from build123d import *

# Parameters (mm, degrees)
SKETCH1_R               = 33
BOSS_EXTRUDE1_DEPTH     = 2
SKETCH5_R               = 27
BOSS_EXTRUDE2_DEPTH     = 2
SKETCH7_W               = 35
SKETCH7_H               = 25
CUT_EXTRUDE2_DEPTH      = 2
FILLET5_R               = 2
CUT_EXTRUDE3_DEPTH      = 47.840153715
CUT_EXTRUDE3_DEPTH_BACK = 47.840153715
SKETCH8_W               = 35
SKETCH8_H               = 5
FILLET3_R               = 2
SKETCH6_R               = 2
CUT_EXTRUDE4_DEPTH      = 10


with BuildPart() as part:
    # Sketch1 → Boss-Extrude1 (new body)
    with BuildSketch(Plane(origin=(0, 0, 0), x_dir=(1, 0, 0), z_dir=(0, 1, 0))):
        with Locations(Location((0, 0, 0), (0, 0, 270))):
            Circle(SKETCH1_R)
    extrude(amount=BOSS_EXTRUDE1_DEPTH)

    # Sketch5 → Boss-Extrude2 (add)
    with BuildSketch(Plane.XZ):
        with Locations(Location((0, 0, 0), (0, 0, 270))):
            Circle(SKETCH5_R)
    extrude(amount=BOSS_EXTRUDE2_DEPTH)

    # Sketch7 → Cut-Extrude2 (cut)
    with BuildSketch(Plane(origin=(0, 2, 0), x_dir=(1, 0, 0), z_dir=(0, 1, 0))):
        Rectangle(SKETCH7_W, SKETCH7_H)
    extrude(amount=-CUT_EXTRUDE2_DEPTH, mode=Mode.SUBTRACT)

    # Fillet5
    fillet5_edges = [part.edges().sort_by_distance(p)[0] for p in [
        (0, -2, 27),
    ]]
    fillet(fillet5_edges, radius=FILLET5_R - 0.0001)  # a hair under: the kernel refuses the full size

    # Sketch8 → Cut-Extrude3 (cut, two sides: drawn at the far end of the back side and taken through both)
    with BuildSketch(Plane(origin=(0, 2, 0), x_dir=(1, 0, 0), z_dir=(0, 1, 0)).offset(-CUT_EXTRUDE3_DEPTH_BACK)):
        with Locations((0, -10)):
            Rectangle(SKETCH8_W, SKETCH8_H)
    extrude(amount=CUT_EXTRUDE3_DEPTH + CUT_EXTRUDE3_DEPTH_BACK, mode=Mode.SUBTRACT)

    # Fillet3
    fillet3_edges = [part.edges().sort_by_distance(p)[0] for p in [
        (0, 2, 12.5),
        (-17.5, 2, 0),
        (0, 2, -12.5),
        (17.5, 2, 0),
    ]]
    fillet(fillet3_edges, radius=FILLET3_R - 0.0001)  # a hair under: the kernel refuses the full size

    # Sketch6 → Cut-Extrude4 (cut)
    with BuildSketch(Plane.XZ):
        with BuildLine():
            ThreePointArc((3.5, 32.813869019), (0, 33), (-3.5, 32.813869019))
            Line((-3.5, 32.813869019), (-2.640595233, 27.71772001))
            ThreePointArc((-2.640595233, 27.71772001), (-2.300161408, 27.12037077), (-1.654518359, 26.884010118))
            Line((-1.654518359, 26.884010118), (1.654518359, 26.884010118))
            ThreePointArc((1.654518359, 26.884010118), (2.300161408, 27.12037077), (2.640595233, 27.71772001))
            Line((2.640595233, 27.71772001), (3.5, 32.813869019))
        make_face()
        with BuildLine():
            Line((25.32454728, 11.572037452), (30.167644167, 13.375845596))
            ThreePointArc((30.167644167, 13.375845596), (28.578838325, 16.5), (26.667644167, 19.438023423))
            Line((26.667644167, 19.438023423), (22.683952047, 16.145682558))
            ThreePointArc((22.683952047, 16.145682558), (22.336849342, 15.552183597), (22.454976538, 14.874859989))
            Line((22.454976538, 14.874859989), (24.109494897, 12.009150128))
            ThreePointArc((24.109494897, 12.009150128), (24.637010751, 11.568187173), (25.32454728, 11.572037452))
        make_face()
        with Locations(Location((-15.850338446, 24.880047651, 0), (0, 0, 270))):
            Circle(SKETCH6_R)
        with BuildLine():
            Line((-30.167644167, 13.375845596), (-25.32454728, 11.572037452))
            ThreePointArc((-25.32454728, 11.572037452), (-24.637010751, 11.568187173), (-24.109494897, 12.009150128))
            Line((-24.109494897, 12.009150128), (-22.454976538, 14.874859989))
            ThreePointArc((-22.454976538, 14.874859989), (-22.336849342, 15.552183597), (-22.683952047, 16.145682558))
            Line((-22.683952047, 16.145682558), (-26.667644167, 19.438023423))
            ThreePointArc((-26.667644167, 19.438023423), (-28.578838325, 16.5), (-30.167644167, 13.375845596))
        make_face()
        with BuildLine():
            Line((22.683952047, -16.145682558), (26.667644167, -19.438023423))
            ThreePointArc((26.667644167, -19.438023423), (28.578838325, -16.5), (30.167644167, -13.375845596))
            Line((30.167644167, -13.375845596), (25.32454728, -11.572037452))
            ThreePointArc((25.32454728, -11.572037452), (24.637010751, -11.568187173), (24.109494897, -12.009150128))
            Line((24.109494897, -12.009150128), (22.454976538, -14.874859989))
            ThreePointArc((22.454976538, -14.874859989), (22.336849342, -15.552183597), (22.683952047, -16.145682558))
        make_face()
        with Locations(Location((15.850338446, -24.880047651, 0), (0, 0, 270))):
            Circle(SKETCH6_R)
        with BuildLine():
            Line((-26.667644167, -19.438023423), (-22.683952047, -16.145682558))
            ThreePointArc((-22.683952047, -16.145682558), (-22.336849342, -15.552183597), (-22.454976538, -14.874859989))
            Line((-22.454976538, -14.874859989), (-24.109494897, -12.009150128))
            ThreePointArc((-24.109494897, -12.009150128), (-24.637010751, -11.568187173), (-25.32454728, -11.572037452))
            Line((-25.32454728, -11.572037452), (-30.167644167, -13.375845596))
            ThreePointArc((-30.167644167, -13.375845596), (-28.578838325, -16.5), (-26.667644167, -19.438023423))
        make_face()
        with BuildLine():
            Line((-2.640595233, -27.71772001), (-3.5, -32.813869019))
            ThreePointArc((-3.5, -32.813869019), (0, -33), (3.5, -32.813869019))
            Line((3.5, -32.813869019), (2.640595233, -27.71772001))
            ThreePointArc((2.640595233, -27.71772001), (2.300161408, -27.12037077), (1.654518359, -26.884010118))
            Line((1.654518359, -26.884010118), (-1.654518359, -26.884010118))
            ThreePointArc((-1.654518359, -26.884010118), (-2.300161408, -27.12037077), (-2.640595233, -27.71772001))
        make_face()
    extrude(amount=-CUT_EXTRUDE4_DEPTH, mode=Mode.SUBTRACT)


solid = part.part
Design review of the part built by this model. Coordinates are the model's own, in mm. A direction names the side the tool comes from. Round coordinates to 2 decimals unless told otherwise and drop trailing zeros. Write each loop counter-clockwise with the first axis right and the second up, starting at its lowest first coordinate (ties: lowest second). Pieces come first, ordered by that corner, then holes. Notation, with made-up numbers: (3.5, 75) -> (11.5, 75) arc R11 ccw to (11.5, 96) -> close; hole circle Ø10 at (48.25, 41.5). An arc over 180 degrees is marked (long way). One line per question, with ' | ' between items.
(1) Take a section at D-D, the plane x = -28. State the section outline as (y, z) points, and give its area (3 significant figures).
Result sheet:
outline: (0, -12.57) -> (2, -12.57) -> (2, 12.57) -> (0, 12.57) -> close | area: 50.3 mm2
(2) Draft analysis for pull direction Z (two halves, no side actions). For faces 1 (the flat face through (0, 2, -15)), 2 (the cylindrical face through (16.67, 0.99, -28.48)), 3 (the flat face through (-24.65, 0.99, 17.77)), 4 (the flat face through (0, -1, 7.5)), state which applies: released by +Z, released by -Z, zero draft, split by the parting line, or undercut.
Result sheet:
face 1: zero draft | face 2: released by -Z | face 3: undercut | face 4: undercut
(3) Machinability: for faces 5 (the flat face through (0, 1, -26.884)), 6 (the flat face through (0, -1, 12.5)), 7 (the flat face through (-3.076, 0.986, 30.301)), 8 (the flat face through (13, 0, -27)), which of the approach directions +Z, -Z, +X, -X, +Y, -Y give a long, thin tool a straight path to every point of the face, cutting with its end or side? Answer none if there is none.
Result sheet:
face 5: -Z, +Y | face 6: +Y, -Y | face 7: +Z, +Y, -Y | face 8: -Z, +X, -Y
(4) Take a section at C-C, the plane y = 0.9. State how many separate pieces and enclosed holes the cut face has, and give its area (3 significant figures).
Result sheet:
separate pieces: 1 | enclosed holes: 3 | area: 2,280 mm2
(5) Wall thickness on line 1 (Y direction, x = -5, z = -28); line 2 (X direction, y = 0.65, z = -30); line 3 (Z direction, x = -1, y = 0.7): over which ranges is each line inside the solid? List them lowest first. Write a range as [from, to].
Result sheet:
line 1: [0, 2] | line 2: [-13.75, -3.03], [3.03, 13.75] | line 3: [-26.88, -12.63], [12.63, 26.88]
(6) Insertion check: P1, Ø16, axis at x = 2.5, z = -5, coming from the +Y side; P2, Ø6, axis at x = 19, z = -21.5, coming from the -Y side; P3, Ø1.6, axis at y = -1, z = 0, coming from the -X side. Each pin has a flat end and moves straight along its axis. Give the tip position at first contact, or say it passes through.
Result sheet:
P1: y = 1.32 | P2: y = -1.88 | P3: x = -26.99
